from build123d import *

# Parameters (mm, degrees)
F3_START = 2
F3_DEPTH = 10.001


with BuildPart() as f1:
    # F0 (on Right) → F1 (revolve)
    with BuildSketch(Plane.YZ):
        with BuildLine():
            Line((-17, 0), (-11.5, 0))
            Line((-11.5, 0), (-11.5, 2))
            Line((-11.5, 2), (-13.25, 2))
            Line((-13.25, 2), (-13.25, 10))
            Line((-13.25, 10), (-13.2623105626, 10))
            ThreePointArc((-13.2623105626, 10), (-12.9470283874, 10.1538351162), (-12.8742535625, 10.49701425))
            Line((-12.8742535625, 10.49701425), (-13.25, 12))
            Line((-13.25, 12), (-17, 12))
            Line((-17, 12), (-15, 10))
            Line((-15, 10), (-15, 2))
            Line((-15, 2), (-17, 0))
        make_face()
    revolve(axis=Axis((0, 0, 6), (0, 0, 1)))

    # F2 (on Top) → F3 (cut)
    with BuildSketch(Plane.XY.offset(F3_START)):
        with BuildLine():
            ThreePointArc((-1, 13.2122102617), (-9.3691648507, 9.3691648507), (-13.2122102617, 1))
            Line((-13.2122102617, 1), (-1, 1))
            Line((-1, 1), (-1, 13.2122102617))
        make_face()
        with BuildLine():
            ThreePointArc((13.2122102617, 1), (9.3691648507, 9.3691648507), (1, 13.2122102617))
            Line((1, 13.2122102617), (1, 1))
            Line((1, 1), (13.2122102617, 1))
        make_face()
        with BuildLine():
            Line((1, -1), (1, -13.2122102617))
            ThreePointArc((1, -13.2122102617), (9.3691648507, -9.3691648507), (13.2122102617, -1))
            Line((13.2122102617, -1), (1, -1))
        make_face()
        with BuildLine():
            Line((-1, -1), (-13.2122102617, -1))
            ThreePointArc((-13.2122102617, -1), (-9.3691648507, -9.3691648507), (-1, -13.2122102617))
            Line((-1, -13.2122102617), (-1, -1))
        make_face()
    extrude(amount=F3_DEPTH, mode=Mode.SUBTRACT)


solid = f1.part
For this review, take the finished solid that the model builds, in its own axes (mm). A direction names the side the tool comes from. Give positions to 0.01 mm unless a question says otherwise; leave off trailing zeros. Loops run counter-clockwise (first coordinate to the right, second up) from the corner with the lowest first, then second, coordinate; pieces in that order, holes last.
Item 1: Insertion check: pin 1 (1.5 mm diameter, centred on x = -7, z = 10.5, fed in from -Y); pin 2 (2 mm diameter, centred on y = -4, z = 10.5, fed in from +X); pin 3 (13 mm diameter, centred on x = -5, y = 3.5, fed in from +Z). Each pin has a flat end and moves straight along its axis. Give the tip position at first contact, or say it passes through.
Item 2: Draft analysis for pull direction Y (two halves, no side actions). For faces 4 (the conical face through (-14.77, 3.28, 1.87)), 5 (the cylindrical face through (-9.46, -9.28, 10.99)), 6 (the flat face through (-9, 10, 12)), state which applies: +Y half, -Y half, draft (parallel to the pull), parting line (faces both ways), or undercut.
Item 3: Take a section at C-C, the plane z = 8. State the section outline as (x, y) points, and give its area (3 significant figures).
Item 4: Tool access review of faces 1 (the cylindrical face through (0.66, 14.985, 5.944)), 2 (the cylindrical face through (11.4, 1.5, 1)), 3 (the conical face through (13, 0, 11)): name each direction out of +Z, -Z, +X, -X, +Y, -Y from which nothing blocks a thin tool from reaching the whole face with its end or side.
Item 5: For line 1 along X through (y, z) = (0, 3.75); line 2 along Z through (x, y) = (-11.5, 12); line 3 along X through (y, z) = (-5, 1.25), list the stretches that pass through material, from the lowest coordinate up.
Calculated:
1. pin 1: stops at y = -14.74
1. pin 2: stops at x = 16.04
1. pin 3: stops at z = 2
2. face 4: parting line
2. face 5: undercut
2. face 6: draft
3. outline: circle Ø30 at (0, 0); hole circle Ø26.5 at (0, 0)
3. area: 155 mm2
4. face 1: none
4. face 2: +Z, -Z
4. face 3: +Z
5. line 1: x = -15 to -13.25, 13.25 to 15
5. line 2: z = 0 to 0.38, 11.62 to 12
5. line 3: x = -14.94 to -10.36, 10.36 to 14.94
